Input: part model. Units: mm. Frame: model coordinates. A direction names the side the tool comes from. Round coordinates to 2 decimals unless told otherwise and drop trailing zeros. Order: outer loops, then holes, each group sorted by start corner. A loop starts at its lowest first (then second) coordinate and runs counter-clockwise, first axis right, second up. Notation, with made-up numbers: (83.5, 28) -> (123.5, 28) arc R29 cw to (123.5, 52) -> close; hole circle Ø3 at (-11.5, 30.25). An arc over 180 degrees is marked (long way). Use a Markdown table: item, result.
from build123d import *

# Parameters (mm, degrees)
SKETCH1_R           = 3.175
BOSS_EXTRUDE1_DEPTH = 3.175
SKETCH2_R           = 11.049
SKETCH2_R_2         = 15.875
SKETCH2_R_3         = 1.27
CUT_EXTRUDE1_DEPTH  = 202.930998425
ITC_CUTOUT_DEPTH    = 202.930998425
SKETCH6_W           = 67.523241089
SKETCH6_H           = 6.35
CUT_EXTRUDE3_DEPTH  = 202.930998425
FILLET1_R           = 6.35
CUT_EXTRUDE4_DEPTH  = 202.930998425
FILLET2_R           = 6.35
SKETCH8_R           = 1.5875
CUT_EXTRUDE5_DEPTH  = 202.930998425
SKETCH10_R          = 1.5875
CUT_EXTRUDE6_DEPTH  = 202.930998425


with BuildPart() as part:
    # Sketch1 → Boss-Extrude1 (new, symmetric)
    with BuildSketch(Plane.XY):
        with BuildLine():
            Line((-145.783553311, 66.675), (145.783553311, 66.675))
            ThreePointArc((145.783553311, 66.675), (147.900219978, 66.497368874), (149.957676269, 65.969444444))
            ThreePointArc((149.957676269, 65.969444444), (172.789871953, 52.74760778), (189.088888889, 31.999880883))
            ThreePointArc((189.088888889, 31.999880883), (190.142181511, 29.17513943), (190.5, 26.181720723))
            Line((190.5, 26.181720723), (190.5, -22.225))
            ThreePointArc((190.5, -22.225), (186.780256121, -31.205256121), (177.8, -34.925))
            Line((177.8, -34.925), (-177.8, -34.925))
            ThreePointArc((-177.8, -34.925), (-186.780256121, -31.205256121), (-190.5, -22.225))
            Line((-190.5, -22.225), (-190.5, 26.181720723))
            ThreePointArc((-190.5, 26.181720723), (-190.142181511, 29.17513943), (-189.088888889, 31.999880883))
            ThreePointArc((-189.088888889, 31.999880883), (-172.789871953, 52.74760778), (-149.957676269, 65.969444444))
            ThreePointArc((-149.957676269, 65.969444444), (-147.900219978, 66.497368874), (-145.783553311, 66.675))
        make_face()
        with Locations((-127, 0)):
            Circle(SKETCH1_R, mode=Mode.SUBTRACT)
        with Locations((127, 0)):
            Circle(SKETCH1_R, mode=Mode.SUBTRACT)
    extrude(amount=BOSS_EXTRUDE1_DEPTH, both=True)

    # Sketch2 → Cut-Extrude1 (cut, through all)
    with BuildSketch(Plane.XY.offset(3.175)):
        with Locations((-127, 0)):
            Circle(SKETCH2_R)
        with Locations((-160.3375, 0)):
            Circle(SKETCH2_R_2)
        with Locations((-143.499519773, 16.837980227)):
            Circle(SKETCH2_R_3)
        with Locations((-160.3375, 23.8125)):
            Circle(SKETCH2_R_3)
        with Locations((-143.499519773, -16.837980227)):
            Circle(SKETCH2_R_3)
        with Locations((-160.3375, -23.8125)):
            Circle(SKETCH2_R_3)
        with Locations((-177.175480227, -16.837980227)):
            Circle(SKETCH2_R_3)
        with Locations((-184.15, 0)):
            Circle(SKETCH2_R_3)
        with Locations((-177.175480227, 16.837980227)):
            Circle(SKETCH2_R_3)
        with Locations((-127, 15.875)):
            Circle(SKETCH2_R_3)
        with Locations((-115.774679849, 11.225320151)):
            Circle(SKETCH2_R_3)
        with Locations((-111.125, 0)):
            Circle(SKETCH2_R_3)
        with Locations((-115.774679849, -11.225320151)):
            Circle(SKETCH2_R_3)
        with Locations((-127, -15.875)):
            Circle(SKETCH2_R_3)
        with Locations((-138.225320151, -11.225320151)):
            Circle(SKETCH2_R_3)
        with Locations(Location((138.225320151, 11.225320151, 0), (0, 0, 180))):
            Circle(SKETCH2_R_3)
        with Locations((-138.225320151, 11.225320151)):
            Circle(SKETCH2_R_3)
        with Locations(Location((138.225320151, -11.225320151, 0), (0, 0, 180))):
            Circle(SKETCH2_R_3)
        with Locations(Location((127, -15.875, 0), (0, 0, 180))):
            Circle(SKETCH2_R_3)
        with Locations(Location((115.774679849, -11.225320151, 0), (0, 0, 180))):
            Circle(SKETCH2_R_3)
        with Locations(Location((111.125, 0, 0), (0, 0, 180))):
            Circle(SKETCH2_R_3)
        with Locations(Location((115.774679849, 11.225320151, 0), (0, 0, 180))):
            Circle(SKETCH2_R_3)
        with Locations(Location((127, 15.875, 0), (0, 0, 180))):
            Circle(SKETCH2_R_3)
        with Locations(Location((177.175480227, 16.837980227, 0), (0, 0, 180))):
            Circle(SKETCH2_R_3)
        with Locations(Location((184.15, 0, 0), (0, 0, 180))):
            Circle(SKETCH2_R_3)
        with Locations(Location((177.175480227, -16.837980227, 0), (0, 0, 180))):
            Circle(SKETCH2_R_3)
        with Locations(Location((160.3375, -23.8125, 0), (0, 0, 180))):
            Circle(SKETCH2_R_3)
        with Locations(Location((143.499519773, -16.837980227, 0), (0, 0, 180))):
            Circle(SKETCH2_R_3)
        with Locations(Location((160.3375, 23.8125, 0), (0, 0, 180))):
            Circle(SKETCH2_R_3)
        with Locations(Location((143.499519773, 16.837980227, 0), (0, 0, 180))):
            Circle(SKETCH2_R_3)
        with Locations(Location((160.3375, 0, 0), (0, 0, 180))):
            Circle(SKETCH2_R_2)
        with Locations(Location((127, 0, 0), (0, 0, 180))):
            Circle(SKETCH2_R)
    extrude(amount=-CUT_EXTRUDE1_DEPTH, mode=Mode.SUBTRACT)

    # Sketch5 → ITC_Cutout (cut, through all)
    with BuildSketch(Plane.XY.offset(3.175)):
        with BuildLine():
            Line((-88.9, 15.875), (88.9, 15.875))
            ThreePointArc((88.9, 15.875), (97.880256121, 19.594743879), (101.6, 28.575))
            Line((101.6, 28.575), (101.6, 66.675))
            Line((101.6, 66.675), (-101.6, 66.675))
            Line((-101.6, 66.675), (-101.6, 28.575))
            ThreePointArc((-101.6, 28.575), (-97.880256121, 19.594743879), (-88.9, 15.875))
        make_face()
    extrude(amount=-ITC_CUTOUT_DEPTH, mode=Mode.SUBTRACT)

    # Sketch6 → Cut-Extrude3 (cut, through all)
    with BuildSketch(Plane.XY.offset(3.175)):
        with Locations((-105.671932766, 63.5)):
            Rectangle(SKETCH6_W, SKETCH6_H)
        with Locations((105.671932766, 63.5)):
            Rectangle(SKETCH6_W, SKETCH6_H)
    extrude(amount=-CUT_EXTRUDE3_DEPTH, mode=Mode.SUBTRACT)

    # Fillet1
    fillet1_edges = [part.edges().sort_by_distance(p)[0] for p in [
        (-101.6, 60.325, 0),
        (101.6, 60.325, 0),
    ]]
    fillet(fillet1_edges, radius=FILLET1_R)

    # Sketch7 → Cut-Extrude4 (cut, through all)
    with BuildSketch(Plane.XY.offset(3.175)):
        with BuildLine():
            Line((-88.9, -15.875), (88.9, -15.875))
            ThreePointArc((88.9, -15.875), (97.880256121, -19.594743879), (101.6, -28.575))
            Line((101.6, -28.575), (101.6, -34.925))
            Line((101.6, -34.925), (-101.6, -34.925))
            Line((-101.6, -34.925), (-101.6, -28.575))
            ThreePointArc((-101.6, -28.575), (-97.880256121, -19.594743879), (-88.9, -15.875))
        make_face()
    extrude(amount=-CUT_EXTRUDE4_DEPTH, mode=Mode.SUBTRACT)

    # Fillet2
    fillet2_edges = [part.edges().sort_by_distance(p)[0] for p in [
        (101.6, -34.925, 0),
        (-101.6, -34.925, 0),
    ]]
    fillet(fillet2_edges, radius=FILLET2_R - 0.0001)  # a hair under: the kernel refuses the full size

    # Sketch8 → Cut-Extrude5 (cut, through all)
    with BuildSketch(Plane.XY.offset(3.175)):
        with Locations((-135.369553311, 53.975)):
            Circle(SKETCH8_R)
        with Locations((-105.524553311, 53.975)):
            Circle(SKETCH8_R)
        with Locations(Location((105.524553311, 53.975, 0), (0, 0, 180))):
            Circle(SKETCH8_R)
        with Locations(Location((135.369553311, 53.975, 0), (0, 0, 180))):
            Circle(SKETCH8_R)
    extrude(amount=-CUT_EXTRUDE5_DEPTH, mode=Mode.SUBTRACT)

    # Sketch10 → Cut-Extrude6 (cut, through all)
    with BuildSketch(Plane.XY.offset(3.175)):
        with Locations((-177.8, -28.575)):
            Circle(SKETCH10_R)
        with Locations((-107.95, -28.575)):
            Circle(SKETCH10_R)
        with Locations(Location((107.95, -28.575, 0), (0, 0, 180))):
            Circle(SKETCH10_R)
        with Locations(Location((177.8, -28.575, 0), (0, 0, 180))):
            Circle(SKETCH10_R)
        Circle(SKETCH10_R)
    extrude(amount=-CUT_EXTRUDE6_DEPTH, mode=Mode.SUBTRACT)


solid = part.part
1) Pin query (flat end, axial travel): pin 1 Ø3 at (y, z) = (64.5, -1.5) entering from +X; pin 2 Ø3 at (x, y) = (105.52, 53.98) entering from -Z; pin 3 Ø1.9 at (x, z) = (122, -0.5) entering from +Y (3 decimals). Return the tip coordinate at first contact, or that it passes through.
Results found:
| item | result |
|---|---|
| pin 1 | stops at x = 157.17 |
| pin 2 | passes through |
| pin 3 | stops at y = 60.325 |
2) Set-up query: faces 5 (the cylindrical face through (-103.509, -33.114, -0.044)), 6 (the flat face through (-139.434, 63, 0)), 7 (the cylindrical face through (138.04, -0.49, 0.04)). Return all of +Z, -Z, +X, -X, +Y, -Y with unobstructed straight access to the full face (end or side cutting, diameter ignored); none if empty.
Results found:
| item | result |
|---|---|
| face 5 | +Z, -Z, -Y |
| face 6 | +Z, -Z, +Y |
| face 7 | +Z, -Z |
3) Cut plane C-C on x = 84.5. Return loops of the section in (y, z) (3 decimals), and give its area (3 significant figures).
Results found:
| item | result |
|---|---|
| outline | (-15.875, -3.175) -> (15.875, -3.175) -> (15.875, 3.175) -> (-15.875, 3.175) -> close |
| area | 202 mm² |
4) Cut plane B-B on z = 1. Count the separate pieces of the cut face and the enclosed holes in it, and give its area (3 significant figures).
Results found:
| item | result |
|---|---|
| separate pieces | 1 |
| enclosed holes | 41 |
| area | 20,400 mm² |
5) Line query: L1, parallel to Y at x = -127, z = -1.5 (3 decimals); L2, parallel to Y at x = -136, z = 0 (3 decimals); L3, parallel to Y at x = -2, z = -2 (3 decimals). Output: solid intervals per line, ascending. Write a range as [from, to].
Results found:
| item | result |
|---|---|
| L1 | y = [-34.925, -17.145], [-14.605, -11.049], [11.049, 14.605], [17.145, 60.325] |
| L2 | y = [-34.925, -6.409], [6.409, 52.518], [55.432, 60.325] |
| L3 | y = [-15.875, 15.875] |
6) Pull-direction query (Y, two-part tool) for faces 1 (the cylindrical face through (172.935, 9.66, 0.044)), 2 (the flat face through (-1, 15.875, 0)), 3 (the cylindrical face through (103.411, -33.016, -0.044)), 4 (the flat face through (3, 5, -3.175)); classes: +Y half, -Y half, draft (parallel to the pull), parting line (faces both ways), or undercut.
Results found:
| item | result |
|---|---|
| face 1 | undercut |
| face 2 | +Y half |
| face 3 | -Y half |
| face 4 | draft |
7) Cut plane A-A on y = 35.5. Return loops of the section in (x, z) (3 decimals), and give its area (3 significant figures).
Results found:
| item | result |
|---|---|
| outline | (-187.156, -3.175) -> (-101.6, -3.175) -> (-101.6, 3.175) -> (-187.156, 3.175) -> close; (101.6, -3.175) -> (187.156, -3.175) -> (187.156, 3.175) -> (101.6, 3.175) -> close |
| area | 1,090 mm² |
